from build123d import *

# Parameters (mm, degrees)
F0_W     = 8.1
F0_H     = 3.1
F1_DEPTH = 10


with BuildPart() as f1:
    # F0 (on Top) → F1 (new body)
    with BuildSketch(Plane.XY):
        with BuildLine():
            ThreePointArc((20.1, -15.834965), (19.22132, -17.956285), (17.1, -18.834965))
            Line((17.1, -18.834965), (-17.1, -18.834965))
            ThreePointArc((-17.1, -18.834965), (-19.22132, -17.956285), (-20.1, -15.834965))
            Line((-20.1, -15.834965), (-20.1, -3))
            ThreePointArc((-20.1, -3), (-20.97868, -0.87868), (-23.1, 0))
            Line((-23.1, 0), (-23.1, -23.637105))
            ThreePointArc((-23.1, -23.637105), (-23.355919, -25.370754), (-24.101846, -26.956511))
            Line((-24.101846, -26.956511), (-32.833091, -40.10347))
            Line((-32.833091, -40.10347), (-24.244918, -40.10347))
            Line((-24.244918, -40.10347), (-22.869062, -38.031792))
            Line((-22.869062, -38.031792), (0, -38.031792))
            Line((0, -38.031792), (22.869062, -38.031792))
            Line((22.869062, -38.031792), (24.244918, -40.10347))
            Line((24.244918, -40.10347), (32.833091, -40.10347))
            Line((32.833091, -40.10347), (24.101846, -26.956511))
            ThreePointArc((24.101846, -26.956511), (23.355919, -25.370754), (23.1, -23.637105))
            Line((23.1, -23.637105), (23.1, 0))
            ThreePointArc((23.1, 0), (20.97868, -0.87868), (20.1, -3))
            Line((20.1, -3), (20.1, -15.834965))
        make_face()
        with Locations((-16.173929, -32.481792)):
            Rectangle(F0_W, F0_H, mode=Mode.SUBTRACT)
        with Locations((16.173929, -32.481792)):
            Rectangle(F0_W, F0_H, mode=Mode.SUBTRACT)
        with BuildLine():
            ThreePointArc((-6.487891, -28.46048), (-5.609211, -26.339159), (-3.487891, -25.46048))
            Line((-3.487891, -25.46048), (3.487891, -25.46048))
            ThreePointArc((3.487891, -25.46048), (5.609211, -26.339159), (6.487891, -28.46048))
            Line((6.487891, -28.46048), (6.487891, -28.74646))
            ThreePointArc((6.487891, -28.74646), (5.609211, -30.86778), (3.487891, -31.74646))
            Line((3.487891, -31.74646), (-3.487891, -31.74646))
            ThreePointArc((-3.487891, -31.74646), (-5.609211, -30.86778), (-6.487891, -28.74646))
            Line((-6.487891, -28.74646), (-6.487891, -28.46048))
        make_face(mode=Mode.SUBTRACT)
    extrude(amount=F1_DEPTH)


solid = f1.part
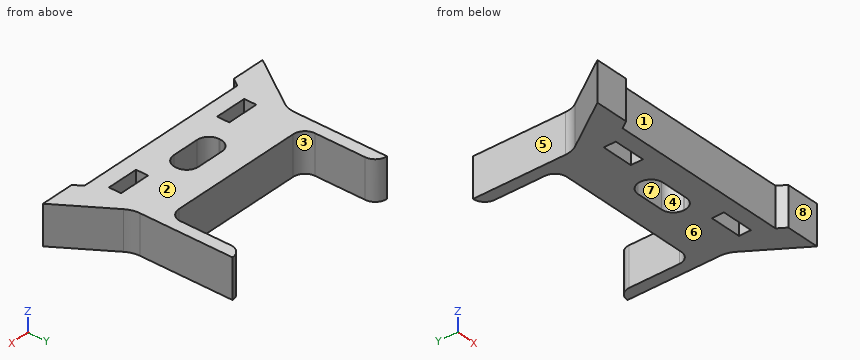
Source: CAD feature listing. Evaluate the final solid. Frame: model axes, mm. Face numbers are marked on the shaded views. A direction names the side the tool comes from. Give positions to 0.01 mm unless a question says otherwise; leave off trailing zeros. Write each loop counter-clockwise with the first axis right and the second up, starting at its lowest first coordinate (ties: lowest second). Pieces come first, ordered by that corner, then holes. Notation, with made-up numbers: M 63,0 L 72,0 A31 ccw 72,35 Z; hole C 19.25,-6 d7. An arc over 180 degrees is marked long. Return JSON: item names as keys, results as strings. Group by question number.
1) Draft query along Y for the marked faces 6, 7 and 8. Return one class per face: released by +Y, released by -Y, zero draft, split by the parting line, or undercut.
2) Cut plane A-A, the plane y = -8. Output: boundary loops of the cut face in (x, z), then the cut area to 3 significant figures.
3) First-contact query: pin 1 Ø3.5 at (x, z) = (-1, 3.5) entering from +Y; pin 2 Ø5 at (y, z) = (-6.5, 5.5) entering from -X; pin 3 Ø8 at (x, y) = (19.5, -8.5) entering from +Z; pin 4 Ø4 at (x, z) = (16, 3) entering from +Y. Flat tips, straight axial feed; report the tip coordinate or a pass-through.
4) Set-up query: the marked faces 1, 2, 3, 4 and 5. Return all of +Z, -Z, +X, -X, +Y, -Y with unobstructed straight access to the full face (end or side cutting, diameter ignored); none if empty.
5) Cut plane D-D, the plane x = 21.5. Output: boundary loops of the cut face in (y, z).
6) Cut plane C-C, the plane z = 1.5. Give the number of separate pieces and of enclosed holes in the cut face, then the cut area to 3 significant figures.
7) Cut plane B-B, the plane x = -13. Output: boundary loops of the cut face in (y, z).
8) Ray query, L1, parallel to X at y = -5, z = 5.75; L2, parallel to Y at x = 16, z = 8.5; L3, parallel to X at y = -33.5, z = 0.5. Return the intervals inside material, ascending.
Data:
{
 "1": {"face 6": "zero draft", "face 7": "undercut", "face 8": "released by -Y"},
 "2": {"outline": "M -23.1,0 L -20.1,0 L -20.1,10 L -23.1,10 Z; M 20.1,0 L 23.1,0 L 23.1,10 L 20.1,10 Z", "area": "60.0 mm²"},
 "3": {"pin 1": "stops at y = -18.83", "pin 2": "stops at x = -23.1", "pin 3": "stops at z = 10", "pin 4": "stops at y = -18.7"},
 "4": {"face 1": "+Z, -Z, -Y", "face 2": "+Z, +X, -X, +Y, -Y", "face 3": "+Z, -Z, +Y", "face 4": "+Z, -Z", "face 5": "+Z, -Z, -X, +Y"},
 "5": {"outline": "M -38.03,0 L -0.46,0 L -0.46,10 L -38.03,10 Z"},
 "6": {"separate pieces": "1", "enclosed holes": "3", "area": "1,020 mm²"},
 "7": {"outline": "M -38.03,0 L -34.03,0 L -34.03,10 L -38.03,10 Z; M -30.93,0 L -18.83,0 L -18.83,10 L -30.93,10 Z"},
 "8": {"L1": "x = -23.1 to -20.1, 20.1 to 23.1", "L2": "y = -38.03 to -34.03, -30.93 to -18.83", "L3": "x = -28.45 to -20.22, -12.12 to 12.12, 20.22 to 28.45"}
}
